```python
from build123d import *

# Parameters (mm, degrees)
SKETCH1_W           = 280
SKETCH1_H           = 65
BOSS_EXTRUDE1_DEPTH = 4
SKETCH2_W           = 4
SKETCH2_H           = 15
CUT_EXTRUDE1_DEPTH  = 4
SKETCH3_W           = 280
SKETCH3_H           = 4
CUT_EXTRUDE2_DEPTH  = 4


with BuildPart() as part:
    # Sketch1 → Boss-Extrude1 (new body)
    with BuildSketch(Plane(origin=(0, 0, 0), x_dir=(1, 0, 0), z_dir=(0, 1, 0))):
        with Locations((140, 32.5)):
            Rectangle(SKETCH1_W, SKETCH1_H)
    extrude(amount=BOSS_EXTRUDE1_DEPTH)

    # Sketch2 → Cut-Extrude1 (cut)
    with BuildSketch(Plane(origin=(0, 4, 0), x_dir=(1, 0, 0), z_dir=(0, 1, 0))):
        with Locations((12, 47.5)):
            Rectangle(SKETCH2_W, SKETCH2_H)
        with Locations((12, 17.5)):
            Rectangle(SKETCH2_W, SKETCH2_H)
        with Locations((72, 17.5)):
            Rectangle(SKETCH2_W, SKETCH2_H)
        with Locations((72, 47.5)):
            Rectangle(SKETCH2_W, SKETCH2_H)
        with Locations((232, 47.5)):
            Rectangle(SKETCH2_W, SKETCH2_H)
        with Locations((232, 17.5)):
            Rectangle(SKETCH2_W, SKETCH2_H)
    extrude(amount=-CUT_EXTRUDE1_DEPTH, mode=Mode.SUBTRACT)

    # Sketch3 → Cut-Extrude2 (cut)
    with BuildSketch(Plane(origin=(0, 4, 0), x_dir=(1, 0, 0), z_dir=(0, 1, 0))):
        with Locations((140, 63)):
            Rectangle(SKETCH3_W, SKETCH3_H)
        with Locations((140, 2)):
            Rectangle(SKETCH3_W, SKETCH3_H)
    extrude(amount=-CUT_EXTRUDE2_DEPTH, mode=Mode.SUBTRACT)


solid = part.part
```
Input: part model. Units: mm. Frame: model coordinates. Coordinates: 2 decimals unless noted, no trailing zeros. Loops run counter-clockwise (first coordinate to the right, second up) from the corner with the lowest first, then second, coordinate; pieces in that order, holes last. Notation, with made-up numbers: (26.5, 47.25) - (52.5, 47.25) arc R20 cw to (52.5, 68.25) - close; hole circle Ø4 at (17, 88.5). An arc over 180 degrees is marked (long way). Answer in a Markdown table with one row per item.
(1) Cut plane B-B on y = 1.3. Output: boundary loops of the cut face in (x, z), plus the area to 3 significant figures.
Model answer:
| item | result |
|---|---|
| outline | (0, -61) - (280, -61) - (280, -4) - (0, -4) - close; hole (10, -55) - (14, -55) - (14, -40) - (10, -40) - close; hole (10, -25) - (14, -25) - (14, -10) - (10, -10) - close; hole (70, -55) - (74, -55) - (74, -40) - (70, -40) - close; hole (70, -25) - (74, -25) - (74, -10) - (70, -10) - close; hole (230, -55) - (234, -55) - (234, -40) - (230, -40) - close; hole (230, -25) - (234, -25) - (234, -10) - (230, -10) - close |
| area | 15,600 mm² |
(2) Cut plane A-A on z = -47. Output: boundary loops of the cut face in (x, y).
Model answer:
| item | result |
|---|---|
| outline | (0, 0) - (10, 0) - (10, 4) - (0, 4) - close; (14, 0) - (70, 0) - (70, 4) - (14, 4) - close; (74, 0) - (230, 0) - (230, 4) - (74, 4) - close; (234, 0) - (280, 0) - (280, 4) - (234, 4) - close |
(3) Material intervals for L1, parallel to X at y = 2.15, z = -42.5; L2, parallel to Z at x = 232.5, y = 0.2, sorted ascending. Write a range as from..to.
Model answer:
| item | result |
|---|---|
| L1 | x = 0..10, 14..70, 74..230, 234..280 |
| L2 | z = -61..-55, -40..-25, -10..-4 |
